Source: three-view drawing plus pictorial views. Frame: mm from the lowest corner of the part. A direction names the side the tool comes from. Give positions to 0.01 mm unless a question says otherwise; leave off trailing zeros. Write each loop counter-clockwise with the first axis right and the second up, starting at its lowest first coordinate (ties: lowest second). Pieces come first, ordered by that corner, then holes.
Q1. Pin query (flat end, axial travel): pin 1 (1 mm diameter, centred on y = 7, z = 5, fed in from +X); pin 2 (3.5 mm diameter, centred on x = 33, y = 7, fed in from -Z); pin 3 (7.5 mm diameter, centred on x = 8, z = 33.5, fed in from +Y); pin 4 (3 mm diameter, centred on x = 7, z = 17, fed in from +Y). Return the tip coordinate at first contact, or that it passes through.
Q2. Line query: L1, parallel to Y at x = 22, z = 10.65; L2, parallel to X at y = 10.5, z = 32.5; L3, parallel to Z at x = 18, y = 4.75. Output: solid intervals per line, ascending.
Q3. Cut plane B-B on y = 1.75. Return the cut outline in (x, z).
Q4. Draft query along Y for the marked faces 4, 5 and 6. Return one class per face: pulls with the +Y half, pulls with the -Y half, needs draft (parallel to the pull), parting line crosses it, or undercut.
Q5. Cut plane C-C on z = 47. Return the cut outline in (x, y).
Q6. Cut plane D-D on x = 37. Return the cut outline in (y, z).
Q7. Reachability of the marked faces 1, 2 and 3 from +Z, -Z, +X, -X, +Y, -Y: full face, straight path, thin tool, end or side. Return the list, or none.
Q8. Cut plane A-A on x = 22. Return the cut outline in (y, z).
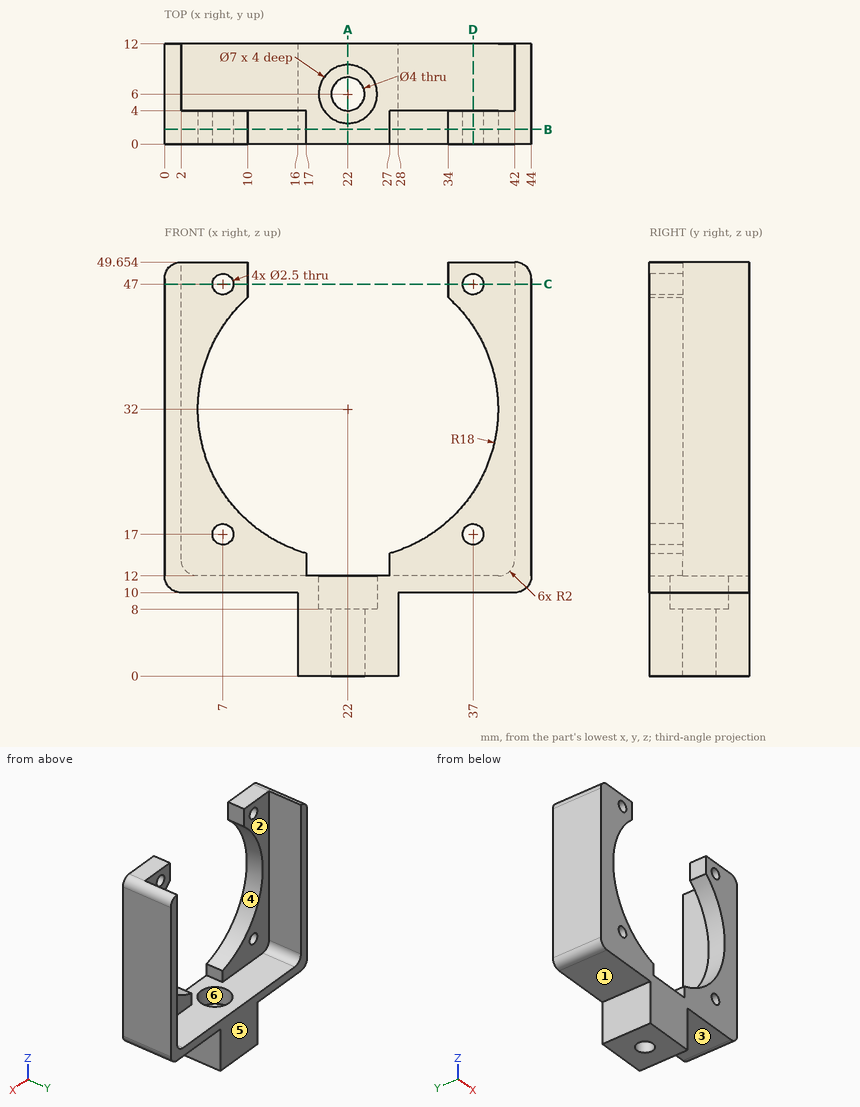
Data:
1. pin 1: stops at x = 28
1. pin 2: stops at z = 10
1. pin 3: passes through
1. pin 4: stops at y = 4
2. L1: y = 0 to 2.5, 9.5 to 12
2. L2: x = 0 to 2, 42 to 44
2. L3: z = 0 to 12
3. outline: (0, 12) arc R2 ccw to (2, 10) - (16, 10) - (16, 0) - (28, 0) - (28, 10) - (42, 10) arc R2 ccw to (44, 12) - (44, 47.65) arc R2 ccw to (42, 49.65) - (34, 49.65) - (34, 45.42) arc R18 cw to (27, 14.71) - (27, 12) - (17, 12) - (17, 14.71) arc R18 cw to (10, 45.42) - (10, 49.65) - (2, 49.65) arc R2 ccw to (0, 47.65) - close; hole circle Ø2.5 at (7, 17); hole circle Ø2.5 at (7, 47); hole circle Ø2.5 at (37, 17); hole circle Ø2.5 at (37, 47)
4. face 4: needs draft
4. face 5: pulls with the +Y half
4. face 6: undercut
5. outline: (0, 0) - (5.75, 0) - (5.75, 4) - (2, 4) - (2, 12) - (0, 12) - close; (8.25, 0) - (10, 0) - (10, 4) - (8.25, 4) - close; (34, 0) - (35.75, 0) - (35.75, 4) - (34, 4) - close; (38.25, 0) - (44, 0) - (44, 12) - (42, 12) - (42, 4) - (38.25, 4) - close
6. outline: (0, 10) - (12, 10) - (12, 12) - (4, 12) - (4, 15.75) - (0, 15.75) - close; (0, 18.25) - (4, 18.25) - (4, 22.05) - (0, 22.05) - close; (0, 41.95) - (4, 41.95) - (4, 45.75) - (0, 45.75) - close; (0, 48.25) - (4, 48.25) - (4, 49.65) - (0, 49.65) - close
7. face 1: -Z, -X, +Y, -Y
7. face 2: +Z, +Y
7. face 3: -Z, +X, +Y, -Y
8. outline: (0, 0) - (4, 0) - (4, 8) - (2.5, 8) - (2.5, 12) - (0, 12) - close; (8, 0) - (12, 0) - (12, 12) - (9.5, 12) - (9.5, 8) - (8, 8) - close
